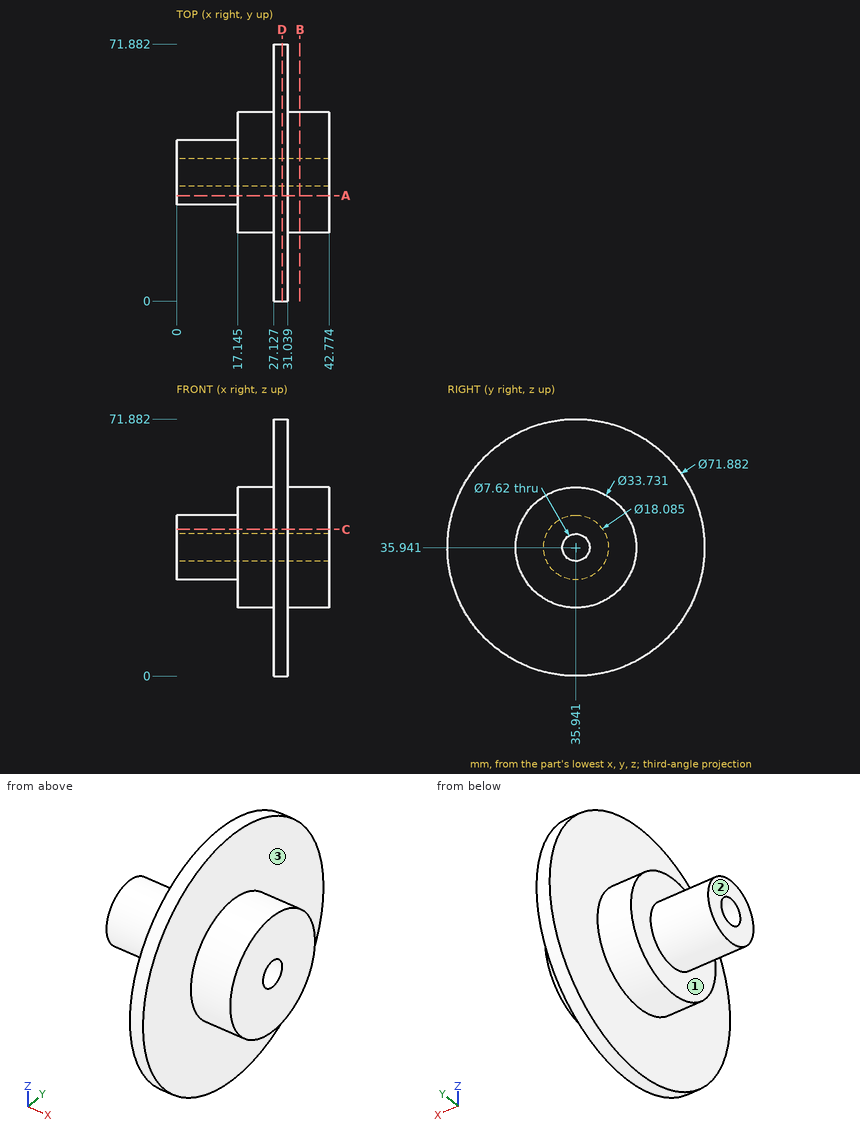
Geometry check sheet. Reference: drawing and pictorial views, mm from the part's lowest x, y, z. A direction names the side the tool comes from. Give positions to 0.01 mm unless a question says otherwise; leave off trailing zeros. Write each loop counter-clockwise with the first axis right and the second up, starting at its lowest first coordinate (ties: lowest second). Pieces come first, ordered by that corner, then holes. Notation, with made-up numbers: (-38, 46.25) - (12, 46.25) arc R17 ccw to (12, 68.25) - close; hole circle Ø8 at (53.5, -31.5). An arc over 180 degrees is marked (long way). Put each result on its own line as item: value.
Q1. Set-up check for the marked faces 1, 2 and 3: record each of +Z, -Z, +X, -X, +Y, -Y from which the full face is reachable in a straight line by a thin tool's end or side.
Result:
face 1: -X
face 2: +Z, -Z, -X, +Y, -Y
face 3: +X
Q2. Section check A-A on y = 29.5. Record the cut outline in (x, z) (1 decimal).
Result:
outline: (0, 29.6) - (17.1, 29.6) - (17.1, 20.4) - (27.1, 20.4) - (27.1, 0.6) - (31, 0.6) - (31, 20.4) - (42.8, 20.4) - (42.8, 51.5) - (31, 51.5) - (31, 71.3) - (27.1, 71.3) - (27.1, 51.5) - (17.1, 51.5) - (17.1, 42.3) - (0, 42.3) - close
Q3. Section check C-C on z = 41. Record the cut outline in (x, y) (1 decimal), and give its area (3 significant figures).
Result:
outline: (0, 28.4) - (17.1, 28.4) - (17.1, 19.9) - (27.1, 19.9) - (27.1, 0.4) - (31, 0.4) - (31, 19.9) - (42.8, 19.9) - (42.8, 52) - (31, 52) - (31, 71.5) - (27.1, 71.5) - (27.1, 52) - (17.1, 52) - (17.1, 43.4) - (0, 43.4) - close
area: 1,230 mm2
Q4. Scan lines: probe 1 along X at (y, z) = (52, 22); probe 2 along Y at (x, z) = (22.5, 36.5) (1 decimal); probe 3 along Y at (x, z) = (29.5, 33.5) (1 decimal). Record each from-to range of solid material in increasing order. Write a range as from..to.
Result:
probe 1: 27.13..31.04
probe 2: 19.1..32.2, 39.7..52.8
probe 3: 0.1..33, 38.9..71.8
Q5. Section check B-B on x = 34.5. Record the cut outline in (y, z) (1 decimal).
Result:
outline: circle Ø33.7 at (35.9, 35.9); hole circle Ø7.6 at (35.9, 35.9)
Q6. Section check D-D on x = 29.5. Record the cut outline in (y, z), and give its area (3 significant figures).
Result:
outline: circle Ø71.88 at (35.94, 35.94); hole circle Ø7.62 at (35.94, 35.94)
area: 4,010 mm2
Q7. Depth check by flat-ended pin: P1, Ø6, axis at y = 51.5, z = 28.5, coming from the -X side (3 decimals); P2, Ø1.5, axis at x = 30, y = 41, coming from the -Z side; P3, Ø5, axis at x = 23.5, y = 64.5, coming from the -Z side; P4, Ø5, axis at x = 32, z = 10.5, coming from the +Y side. Enter the tip coordinate at first touch or a pass-through.
Result:
P1: x = 17.145
P2: z = 0.26
P3: through
P4: y = 63.45
